Job drawing, mm, ordinate dimensions from the low corner. One solid piece. Coordinates: 2 decimals unless noted, no trailing zeros. Write each loop counter-clockwise with the first axis right and the second up, starting at its lowest first coordinate (ties: lowest second). Pieces come first, ordered by that corner, then holes. Notation, with made-up numbers: M 30.5,83.25 L 49.5,83.25 A37 cw 49.5,119.25 Z; hole C 45.5,-14.5 d5. An arc over 180 degrees is marked long. Answer as CSV lines item,"result". Start each with the question number.
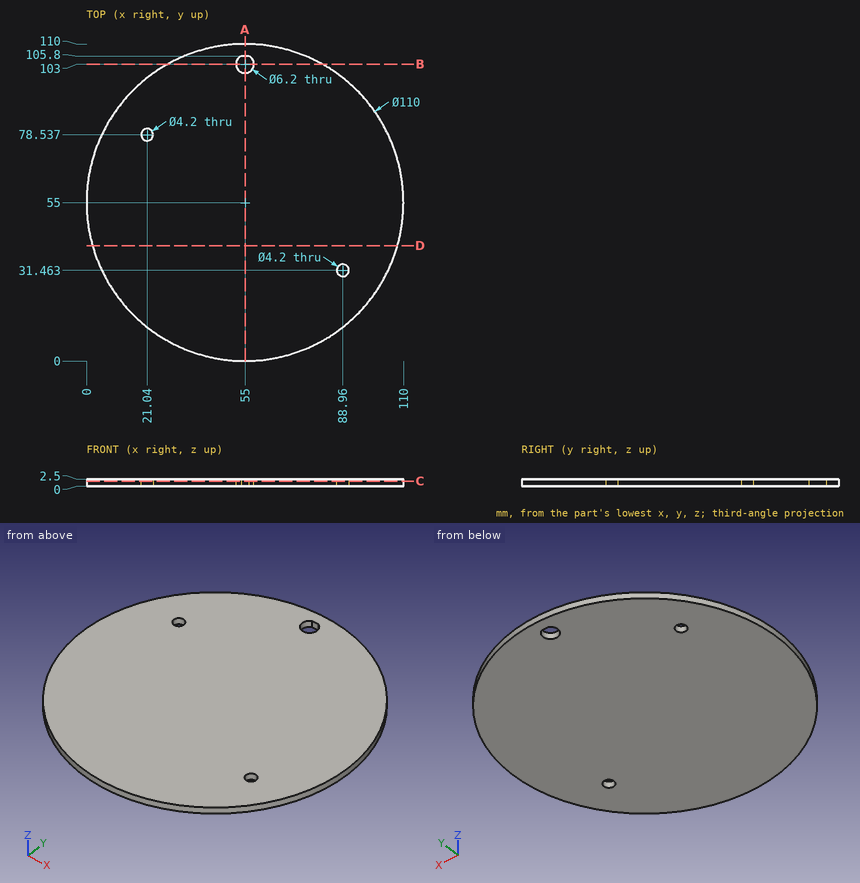
1) Band-saw the part on B-B, the plane y = 103. List the corners of the cut face in (x, z), plus the area to 3 significant figures.
2) Band-saw the part on A-A, the plane x = 55. List the corners of the cut face in (y, z).
3) Pin check, flat tips, straight feed: P1, Ø1, axis at x = 22, z = 1.5, coming from the -Y side; P2, Ø1.2, axis at x = 54.5, z = 1.5, coming from the -Y side; P3, Ø1.5, axis at y = 33, z = 1, coming from the -X side. Stop position of each tip, or through.
4) Probe L1, parallel to X at y = 105, z = 1 (1 decimal); L2, parallel to Y at x = 22.5, z = 1.05 (1 decimal); L3, parallel to X at y = 101.5, z = 2 (1 decimal). List the from-to ranges inside material, lowest first. Write a range as [from, to].
5) Band-saw the part on D-D, the plane y = 40. List the corners of the cut face in (x, z) (1 decimal).
6) Band-saw the part on C-C, the plane z = 1.75. List the corners of the cut face in (x, y), plus the area to 3 significant figures.
Result sheet:
1,outline,"M 28.15,0 L 51.9,0 L 51.9,2.5 L 28.15,2.5 Z; M 58.1,0 L 81.85,0 L 81.85,2.5 L 58.1,2.5 Z"
1,area,"119 mm²"
2,outline,"M 0,0 L 99.9,0 L 99.9,2.5 L 0,2.5 Z; M 105.8,0 L 110,0 L 110,2.5 L 105.8,2.5 Z"
3,P1,"stops at y = 10.63"
3,P2,"stops at y = 0"
3,P3,"stops at x = 4.27"
4,L1,"x = [32.1, 52.6], [57.4, 77.9]"
4,L2,"y = [10.6, 77], [80, 99.4]"
4,L3,"x = [25.6, 52.3], [57.7, 84.4]"
5,outline,"M 2.1,0 L 107.9,0 L 107.9,2.5 L 2.1,2.5 Z"
6,outline,"C 55,55 d110; hole C 21.04,78.54 d4.2; hole M 53.67,105.8 A3.1 ccw long 56.33,105.8 Z; hole C 88.96,31.46 d4.2"
6,area,"9,450 mm²"
